For this review, take the finished solid that the model builds, in its own axes (mm). Face numbers are marked on the shaded views. Give positions to 0.01 mm unless a question says otherwise; leave off trailing zeros. Write each loop counter-clockwise with the first axis right and the second up, starting at its lowest first coordinate (ties: lowest second). Pieces come first, ordered by that corner, then holes.
1) Wall thickness on line 1 along Y through (x, z) = (27.25, -2.5); line 2 along Z through (x, y) = (24, 11.5); line 3 along X through (y, z) = (6.5, -26): over which ranges is each line inside the solid? List them lowest first.
2) We need section D-D on z = -24.5. Give the boundary of the cut face in (x, y).
3) For P1, Ø6.5, axis at x = 28.5, y = -27, coming from the -Z side; P2, Ø4, axis at x = -26, z = -12.5, coming from the +Y side; P3, Ø0.9, axis at x = 29, z = -1.5, coming from the +Y side; P4, Ø8, axis at y = -17.5, z = -3, coming from the +X side, all flat-tipped, find the tip position at first contact; note any pin that passes through.
4) Draft analysis for pull direction Y (two halves, no side actions). For the marked faces 1, 2 and 3, state which applies: pulls with the +Y half, pulls with the -Y half, needs draft (parallel to the pull), parting line crosses it, or undercut.
5) We need section C-C on z = -1.5. Give the boundary of the cut face in (x, y).
6) We need section A-A on y = 0. Give the boundary of the cut face in (x, z), and give its area (3 significant figures).
7) We need section B-B on x = 0. Give the boundary of the cut face in (y, z), and give its area (3 significant figures).
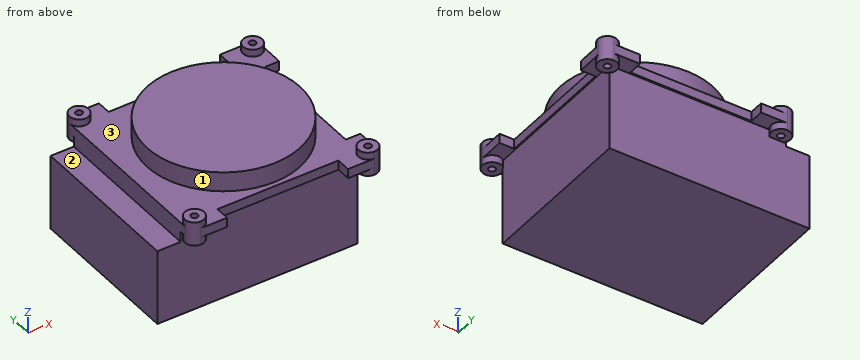
from build123d import *

# Parameters (mm, degrees)
F0_R      = 24
F1_DEPTH  = 6.15
F0_R_2    = 1.05
F2_DEPTH  = 2.25
F3_DEPTH  = 5.3
F4_DEPTH  = 3
F6_W      = 55.5
F6_H      = 50
F7_DEPTH  = 30
F9_W      = 50
F9_H      = 23.7
F10_DEPTH = 7.3


with BuildPart() as f1:
    # F0 (on Top) → F1 (new body)
    with BuildSketch(Plane.XY):
        Circle(F0_R)
    extrude(amount=F1_DEPTH)


with BuildPart() as f2:
    # F0 (on Top) → F2 (new body)
    with BuildSketch(Plane.XY):
        with BuildLine():
            ThreePointArc((27.25, -30), (29.37132, -29.12132), (30.25, -27))
            ThreePointArc((30.25, -27), (25.12868, -24.87868), (27.25, -30))
        make_face()
        with Locations((27.25, -27)):
            Circle(F0_R_2, mode=Mode.SUBTRACT)
        with BuildLine():
            ThreePointArc((30.25, 27), (29.37132, 29.12132), (27.25, 30))
            ThreePointArc((27.25, 30), (25.12868, 24.87868), (30.25, 27))
        make_face()
        with Locations((27.25, 27)):
            Circle(F0_R_2, mode=Mode.SUBTRACT)
        with BuildLine():
            ThreePointArc((-24.25, 27), (-25.12868, 29.12132), (-27.25, 30))
            ThreePointArc((-27.25, 30), (-29.37132, 29.12132), (-30.25, 27))
            ThreePointArc((-30.25, 27), (-27.25, 24), (-24.25, 27))
        make_face()
        with Locations((-27.25, 27)):
            Circle(F0_R_2, mode=Mode.SUBTRACT)
        with BuildLine():
            ThreePointArc((-24.25, -27), (-27.25, -24), (-30.25, -27))
            ThreePointArc((-30.25, -27), (-29.37132, -29.12132), (-27.25, -30))
            ThreePointArc((-27.25, -30), (-25.12868, -29.12132), (-24.25, -27))
        make_face()
        with Locations((-27.25, -27)):
            Circle(F0_R_2, mode=Mode.SUBTRACT)
    extrude(amount=F2_DEPTH)


with BuildPart() as f3:
    # F0 (on Top) → F3 (new body)
    with BuildSketch(Plane.XY):
        with BuildLine():
            ThreePointArc((-24.25, -27), (-27.25, -24), (-30.25, -27))
            ThreePointArc((-30.25, -27), (-29.37132, -29.12132), (-27.25, -30))
            ThreePointArc((-27.25, -30), (-25.12868, -29.12132), (-24.25, -27))
        make_face()
        with Locations((-27.25, -27)):
            Circle(F0_R_2, mode=Mode.SUBTRACT)
        with BuildLine():
            ThreePointArc((-24.25, 27), (-25.12868, 29.12132), (-27.25, 30))
            ThreePointArc((-27.25, 30), (-29.37132, 29.12132), (-30.25, 27))
            ThreePointArc((-30.25, 27), (-27.25, 24), (-24.25, 27))
        make_face()
        with Locations((-27.25, 27)):
            Circle(F0_R_2, mode=Mode.SUBTRACT)
        with BuildLine():
            ThreePointArc((27.25, -30), (29.37132, -29.12132), (30.25, -27))
            ThreePointArc((30.25, -27), (25.12868, -24.87868), (27.25, -30))
        make_face()
        with Locations((27.25, -27)):
            Circle(F0_R_2, mode=Mode.SUBTRACT)
        with BuildLine():
            ThreePointArc((30.25, 27), (29.37132, 29.12132), (27.25, 30))
            ThreePointArc((27.25, 30), (25.12868, 24.87868), (30.25, 27))
        make_face()
        with Locations((27.25, 27)):
            Circle(F0_R_2, mode=Mode.SUBTRACT)
    extrude(amount=-F3_DEPTH)


with BuildPart() as f4:
    # F0 (on Top) → F4 (new body)
    with BuildSketch(Plane.XY):
        with BuildLine():
            ThreePointArc((30.25, 27), (25.12868, 24.87868), (27.25, 30))
            Line((27.25, 30), (19, 30))
            Line((19, 30), (19, 25.5))
            Line((19, 25.5), (-19, 25.5))
            Line((-19, 25.5), (-19, 30))
            Line((-19, 30), (-27.25, 30))
            ThreePointArc((-27.25, 30), (-25.12868, 29.12132), (-24.25, 27))
            ThreePointArc((-24.25, 27), (-27.25, 24), (-30.25, 27))
            Line((-30.25, 27), (-30.25, -27))
            ThreePointArc((-30.25, -27), (-27.25, -24), (-24.25, -27))
            ThreePointArc((-24.25, -27), (-25.12868, -29.12132), (-27.25, -30))
            Line((-27.25, -30), (-19, -30))
            Line((-19, -30), (-19, -25.5))
            Line((-19, -25.5), (19, -25.5))
            Line((19, -25.5), (19, -30))
            Line((19, -30), (27.25, -30))
            ThreePointArc((27.25, -30), (25.12868, -24.87868), (30.25, -27))
            Line((30.25, -27), (30.25, -19))
            Line((30.25, -19), (25.65, -19))
            Line((25.65, -19), (25.65, 19))
            Line((25.65, 19), (30.25, 19))
            Line((30.25, 19), (30.25, 27))
        make_face()
        Circle(F0_R, mode=Mode.SUBTRACT)
    extrude(amount=-F4_DEPTH)

    # F5: union F3, F2, F1
    add(f3.part)
    add(f2.part)
    add(f1.part)


with BuildPart() as f7:
    # F6 (on face) → F7 (new body)
    with BuildSketch(Plane.XY):
        with Locations((-2.5, 0)):
            Rectangle(F6_W, F6_H)
    extrude(amount=-F7_DEPTH)


with BuildPart() as f4_1:
    add(f4.part)

    # F8: union F7
    add(f7.part)

    # F9 (on face) → F10 (join)
    with BuildSketch(Plane(origin=(-30.25, 0, 0), x_dir=(0, -1, 0), z_dir=(-1, 0, 0))):
        with Locations((0, -18.15)):
            Rectangle(F9_W, F9_H)
    extrude(amount=F10_DEPTH)


solid = f4_1.part
Results list:
1. line 1: y = -30 to -28.05, -25.95 to -19, 19 to 25.95, 28.05 to 30
1. line 2: z = -30 to 0
1. line 3: x = -37.55 to 25.25
2. outline: (-37.55, -25) - (25.25, -25) - (25.25, 25) - (-37.55, 25) - close
3. P1: stops at z = -5.3
3. P2: stops at y = 25
3. P3: stops at y = 29.7
3. P4: stops at x = 30.25
4. face 1: parting line crosses it
4. face 2: needs draft
4. face 3: undercut
5. outline: (-30.25, -27) arc R3 ccw to (-27.25, -30) - (-19, -30) - (-19, -25.5) - (19, -25.5) - (19, -30) - (27.25, -30) arc R3 ccw to (30.25, -27) - (30.25, -19) - (25.65, -19) - (25.65, 19) - (30.25, 19) - (30.25, 27) arc R3 ccw to (27.25, 30) - (19, 30) - (19, 25.5) - (-19, 25.5) - (-19, 30) - (-27.25, 30) arc R3 ccw to (-30.25, 27) - close; hole circle Ø2.1 at (-27.25, -27); hole circle Ø2.1 at (-27.25, 27); hole circle Ø2.1 at (27.25, -27); hole circle Ø2.1 at (27.25, 27)
6. outline: (-37.55, -30) - (25.25, -30) - (25.25, -3) - (25.65, -3) - (25.65, 0) - (24, 0) - (24, 6.15) - (-24, 6.15) - (-24, 0) - (-30.25, 0) - (-30.25, -6.3) - (-37.55, -6.3) - close
6. area: 2,130 mm2
7. outline: (-25.5, -3) - (-25, -3) - (-25, -30) - (25, -30) - (25, -3) - (25.5, -3) - (25.5, 0) - (24, 0) - (24, 6.15) - (-24, 6.15) - (-24, 0) - (-25.5, 0) - close
7. area: 1,800 mm2
